Autodesk Inventor part; units mm, degrees
ref_plane "YZ Plane" through (0, 0, 0) normal (1, 0, 0) x (0, 1, 0)
ref_plane "XZ Plane" through (0, 0, 0) normal (0, 1, 0) x (-1, 0, 0)
ref_plane "XY Plane" through (0, 0, 0) normal (0, 0, 1) x (1, 0, 0)
sketch "Sketch1" plane through (0, 0, 0) normal (0, 1, 0) x (-1, 0, 0)
  line L0 (0, 0) -> (-22, 0)
  line L1 (-22, 0) -> (-22, -20)
  line L2 (-22, -20) -> (0, -20)
  line L3 (0, -20) -> (0, 0)
  line L4 (-12, -20) -> (-12, 0)
  point P0 (-17, -10)
  point P1 (-22, -10)
  point P2 (-6, -10)
  point P3 (0, -10)
  dimension "d0" = 20
  dimension "d5" = 12
  dimension "d7" = 5
  dimension "d8" = 5
  dimension "d25" = 6
extrude "Extrusion1" add sketch "Sketch1" against normal blind 4
hole "Hole2" at (6, 0, -10) direction (0, -1, 0) diameter 3.4036 end through all
sketch "Sketch3" plane through (0, -4, 0) normal (0, -1, 0) x (1, 0, 0)
  circle A0 centre (6, -10) radius 1.7018 construction
  line L0 (9.1754, -10) -> (7.5877, -12.75)
  line L1 (7.5877, -12.75) -> (4.4123, -12.75)
  line L2 (4.4123, -12.75) -> (2.8246, -10)
  line L3 (2.8246, -10) -> (4.4123, -7.25)
  line L4 (4.4123, -7.25) -> (7.5877, -7.25)
  line L5 (7.5877, -7.25) -> (9.1754, -10)
  dimension "d33" = 5.5
extrude "Extrusion4" cut sketch "Sketch3" against normal blind 2.2
extrude "Extrusion2" add sketch "Sketch1" along normal blind 4 contours L4 L2 L1 L0
sketch "Sketch2" plane through (0, 4, 0) normal (0, 1, 0) x (1, 0, 0)
  point P0 (17, 10)
hole "Hole1" at (17, 4, -10) direction (0, -1, 0) diameter 3.4036 end through all counterbore diameter 6.5024 counterbore depth 2.9972
chamfer "Chamfer1" distance 0.6 angle 45 18 edges at (6, 0, -20) (12, 2, -20) (17, 4, -20) (22, 4, -10) (17, 4, 0) (12, 2, 0) (6, 0, 0) (0, -2, 0) (22, 0, 0) (22, 0, -20) (11, -4, -20) (22, -4, -10) (11, -4, 0) (0, -4, -10) (0, -2, -20) (17, 4, -13.2512) (0, 0, -10) (12, 4, -10)
Geometry: final body of the model. Coordinates: model frame, mm. A direction names the side the tool comes from. Coordinates: 2 decimals unless noted, no trailing zeros. Loops run counter-clockwise (first coordinate to the right, second up) from the corner with the lowest first, then second, coordinate; pieces in that order, holes last. Notation, with made-up numbers: (13, 42.5) -> (23, 42.5) arc R15 cw to (23, 65.5) -> close; hole circle Ø7 at (79.25, 88). An arc over 180 degrees is marked (long way). Use a Markdown table: item, result. Add a question column.
(1) Section query B-B, the plane y = -1. Return loops of the section in (x, z), plus the area to 3 significant figures.
(2) Line query: line 1 along X through (y, z) = (-0.75, -10); line 2 along X through (y, z) = (1.9, -10); line 3 along Z through (x, y) = (6, -0.9). Output: solid intervals per line, ascending.
(3) Section query A-A, the plane x = 17. Return loops of the section in (y, z).
(4) Mould query, pull axis Z, two halves, no side actions, for faces 4 (the cylindrical face through (13.776, 2.185, -10.423)), 5 (the flat face through (12, 2, -10)), 6 (the flat face through (13, -1, 0)), 7 (the flat face through (3.61, -2.92, -8.64)). Classes: pulls with the +Z half, pulls with the -Z half, needs draft (parallel to the pull), parting line crosses it, or undercut.
(5) Section query C-C, the plane y = 2.25. Return loops of the section in (x, z), plus the area to 3 significant figures.
(6) Section query D-D, the plane z = -1.25. Return loops of the section in (x, y), plus the area to 3 significant figures.
(7) Pin query (flat end, axial travel): pin 1 Ø3 at (x, z) = (6, -10) entering from +Y; pin 2 Ø2.5 at (y, z) = (1, -10) entering from -X; pin 3 Ø4.5 at (x, z) = (17, -10) entering from +Y. Return the tip coordinate at first contact, or that it passes through.
(8) Access query for faces 1 (the flat face through (6, 0, -8)), 2 (the flat face through (18.4, 1.003, -8.6)), 3 (the flat face through (8.37, -2.915, -8.606)). Directions: +Z, -Z, +X, -X, +Y, -Y. A direction counts if a zero-diameter tool reaches every point of the face in a straight line with its end or side. Return the directions, or none.
Answer:
| question | item | result |
|---|---|---|
| 1 | outline | (0, -19.4) -> (0.6, -20) -> (21.4, -20) -> (22, -19.4) -> (22, -0.6) -> (21.4, 0) -> (0.6, 0) -> (0, -0.6) -> close; hole circle Ø3.4 at (6, -10); hole circle Ø3.4 at (17, -10) |
| 1 | area | 421 mm^2 |
| 2 | line 1 | x = 0 to 4.3, 7.7 to 15.3, 18.7 to 22 |
| 2 | line 2 | x = 12 to 13.75, 20.25 to 22 |
| 2 | line 3 | z = -20 to -11.7, -8.3 to 0 |
| 3 | outline | (-4, -19.4) -> (-3.4, -20) -> (3.4, -20) -> (4, -19.4) -> (4, -13.85) -> (3.4, -13.25) -> (1, -13.25) -> (1, -11.7) -> (-4, -11.7) -> close; (-4, -8.3) -> (1, -8.3) -> (1, -6.75) -> (3.4, -6.75) -> (4, -6.15) -> (4, -0.6) -> (3.4, 0) -> (-3.4, 0) -> (-4, -0.6) -> close |
| 4 | face 4 | undercut |
| 4 | face 5 | needs draft |
| 4 | face 6 | pulls with the +Z half |
| 4 | face 7 | undercut |
| 5 | outline | (12, -19.4) -> (12.6, -20) -> (21.4, -20) -> (22, -19.4) -> (22, -0.6) -> (21.4, 0) -> (12.6, 0) -> (12, -0.6) -> close; hole circle Ø6.5 at (17, -10) |
| 5 | area | 166 mm^2 |
| 6 | outline | (0, -3.4) -> (0.6, -4) -> (21.4, -4) -> (22, -3.4) -> (22, 3.4) -> (21.4, 4) -> (12.6, 4) -> (12, 3.4) -> (12, 0) -> (0.6, 0) -> (0, -0.6) -> close |
| 6 | area | 127 mm^2 |
| 7 | pin 1 | passes through |
| 7 | pin 2 | stops at x = 0.35 |
| 7 | pin 3 | stops at y = 1 |
| 8 | face 1 | +Z, -Z, -X, +Y |
| 8 | face 2 | +Y |
| 8 | face 3 | -Y |
